from build123d import *

# Parameters (mm, degrees)
CROQUIS1_R              = 1.5
SALIENTE_EXTRUIR1_DEPTH = 1.5


with BuildPart() as part:
    # Croquis1 → Saliente-Extruir1 (new body)
    with BuildSketch(Plane.XY):
        with BuildLine():
            Line((-38.589251844, 20.8), (49.410748156, 20.8))
            ThreePointArc((49.410748156, 20.8), (53.653388843, 19.042640687), (55.410748156, 14.8))
            Line((55.410748156, 14.8), (55.410748156, -21.2))
            ThreePointArc((55.410748156, -21.2), (53.653388843, -25.442640687), (49.410748156, -27.2))
            Line((49.410748156, -27.2), (-38.589251844, -27.2))
            ThreePointArc((-38.589251844, -27.2), (-42.831892531, -25.442640687), (-44.589251844, -21.2))
            Line((-44.589251844, -21.2), (-44.589251844, 14.8))
            ThreePointArc((-44.589251844, 14.8), (-42.831892531, 19.042640687), (-38.589251844, 20.8))
        make_face()
        with Locations((-42.089251844, 13.05)):
            Circle(CROQUIS1_R, mode=Mode.SUBTRACT)
        with Locations((-42.089251844, -19.45)):
            Circle(CROQUIS1_R, mode=Mode.SUBTRACT)
        with Locations((52.910748156, -19.45)):
            Circle(CROQUIS1_R, mode=Mode.SUBTRACT)
        with Locations((52.910748156, 13.05)):
            Circle(CROQUIS1_R, mode=Mode.SUBTRACT)
    extrude(amount=SALIENTE_EXTRUIR1_DEPTH)


solid = part.part
For this review, take the finished solid that the model builds, in its own axes (mm). Round coordinates to 2 decimals unless told otherwise and drop trailing zeros. Loops run counter-clockwise (first coordinate to the right, second up) from the corner with the lowest first, then second, coordinate; pieces in that order, holes last. Notation, with made-up numbers: (-2.5, 43.25) - (40.5, 43.25) arc R27 cw to (40.5, 63.25) - close; hole circle Ø2 at (-29, 14). An arc over 180 degrees is marked (long way). One line per item, written item: value. Start each with the question number.
Item 1: Clearance check with a flat-ended pin moving along its axis: pin 1 Ø2.5 at (x, y) = (-42.09, 13.05) entering from +Z. State where the tip first meets the part, or that it passes through.
Item 2: The part is to be moulded in two halves that separate along Y. For faces 1 (the cylindrical face through (53.7, -25.396, 0.74)), 2 (the flat face through (6, -3, 1.5)), 3 (the cylindrical face through (51.72, 12.14, 0.74)), say which applies: +Y half, -Y half, draft (parallel to the pull), parting line (faces both ways), or undercut.
Item 3: Take a section at A-A (y = 13.05). Give the boundary of the cut face in (x, z).
Item 4: For L1, parallel to X at y = 13, z = 1.1; L2, parallel to X at y = -18.5, z = 1; L3, parallel to X at y = -22.5, z = 0.85, list the stretches that pass through material, from the lowest coordinate up.
Answer below:
1. pin 1: passes through
2. face 1: -Y half
2. face 2: draft
2. face 3: undercut
3. outline: (-44.59, 0) - (-43.59, 0) - (-43.59, 1.5) - (-44.59, 1.5) - close; (-40.59, 0) - (51.41, 0) - (51.41, 1.5) - (-40.59, 1.5) - close; (54.41, 0) - (55.41, 0) - (55.41, 1.5) - (54.41, 1.5) - close
4. L1: x = -44.59 to -43.59, -40.59 to 51.41, 54.41 to 55.41
4. L2: x = -44.59 to -43.25, -40.93 to 51.75, 54.07 to 55.41
4. L3: x = -44.45 to 55.27
